Design review of the part built by this model. Coordinates are the model's own, in mm. A direction names the side the tool comes from. Round coordinates to 2 decimals unless told otherwise and drop trailing zeros. Loops run counter-clockwise (first coordinate to the right, second up) from the corner with the lowest first, then second, coordinate; pieces in that order, holes last. Notation, with made-up numbers: (-33.75, -33.5) - (25.25, -33.5) arc R13 cw to (25.25, -13.5) - close; hole circle Ø5 at (-2, 28). An arc over 180 degrees is marked (long way). Answer as CSV lines item,"result". Start each with the question number.
(1) Mouldability with a two-part tool opening along X and no side actions: class faces 1 (the cylindrical face through (-0.46, 57.47, 0.74)), 2 (the cylindrical face through (17.14, 55.1, 0.74)), 3 (the cylindrical face through (0.1, 61.5, 0.7)) as released by +X, released by -X, zero draft, split by the parting line, or undercut.
(2) Consider section C-C (x = -2). Give the boundary of the cut face in (y, z), and give its area (3 significant figures).
(3) Wall thickness on L1, parallel to X at y = 47, z = 0.65; L2, parallel to X at y = -15, z = 1.2; L3, parallel to X at y = 40.5, z = 0.5: over which ranges is each line inside the solid? List them lowest first.
(4) Consider section B-B (y = -15.25). Give the boundary of the cut face in (x, z), and give its area (3 significant figures).
(5) Consider section A-A (y = -52). Give the boundary of the cut face in (x, z).
(6) Consider section D-D (z = 0.55). Count the separate pieces of the cut face and the enclosed holes in it, and give its area (3 significant figures).
(7) For P1, Ø0.8, axis at y = -44, z = 0.5, coming from the +X side, flat-tipped, find the tip position at first contact; note if it passes through.
(8) For faces 4 (the cylindrical face through (14.175, 50.536, 0.74)), 5 (the cylindrical face through (9.86, -55.1, 0.74)), list the 3-axis set-ups (+Z, -Z, +X, -X, +Y, -Y) from which the entire face can be reached by the end or side of a thin tool; tool diameter is ignored.
from build123d import *

# Parameters (mm, degrees)
F0_R     = 1.5
F0_R_2   = 3.5
F1_DEPTH = 1.5
F3_DEPTH = 1.501
F5_DEPTH = 1.501
F6_R     = 5


with BuildPart() as f1:
    # F0 (on Top) → F1 (new body)
    with BuildSketch(Plane.XY):
        with BuildLine():
            Line((-9.233093, 56), (-15, 56))
            ThreePointArc((-15, 56), (-17.12132, 55.12132), (-18, 53))
            Line((-18, 53), (-18, 38.214102))
            Line((-18, 38.214102), (-20, 34.75))
            Line((-20, 34.75), (-20, -34.75))
            Line((-20, -34.75), (-18, -38.214102))
            Line((-18, -38.214102), (-18, -53))
            ThreePointArc((-18, -53), (-17.12132, -55.12132), (-15, -56))
            Line((-15, -56), (-12, -56))
            ThreePointArc((-12, -56), (-9.87868, -55.12132), (-9, -53))
            Line((-9, -53), (-9, -48))
            ThreePointArc((-9, -48), (-6.363961, -41.636039), (0, -39))
            ThreePointArc((0, -39), (6.363961, -41.636039), (9, -48))
            Line((9, -48), (9, -53))
            ThreePointArc((9, -53), (9.87868, -55.12132), (12, -56))
            Line((12, -56), (15, -56))
            ThreePointArc((15, -56), (17.12132, -55.12132), (18, -53))
            Line((18, -53), (18, -38.214102))
            Line((18, -38.214102), (20, -34.75))
            Line((20, -34.75), (20, 34.75))
            Line((20, 34.75), (18, 38.214102))
            Line((18, 38.214102), (18, 53))
            ThreePointArc((18, 53), (17.12132, 55.12132), (15, 56))
            Line((15, 56), (9.233093, 56))
            ThreePointArc((9.233093, 56), (7.697794, 56.422626), (6.595066, 57.571429))
            ThreePointArc((6.595066, 57.571429), (0, 61.5), (-6.595066, 57.571429))
            ThreePointArc((-6.595066, 57.571429), (-7.697794, 56.422626), (-9.233093, 56))
        make_face()
        with Locations((-13.5, -52)):
            Circle(F0_R, mode=Mode.SUBTRACT)
        with Locations((-15.25, -15.25)):
            Circle(F0_R, mode=Mode.SUBTRACT)
        with Locations((13.5, -52)):
            Circle(F0_R, mode=Mode.SUBTRACT)
        with Locations((15.25, -15.25)):
            Circle(F0_R, mode=Mode.SUBTRACT)
        with Locations((-15.25, 15.25)):
            Circle(F0_R, mode=Mode.SUBTRACT)
        with BuildLine():
            Line((-15, 27), (-15, 30))
            ThreePointArc((-15, 30), (-14, 31), (-13, 30))
            Line((-13, 30), (-13, 27))
            ThreePointArc((-13, 27), (-14, 26), (-15, 27))
        make_face(mode=Mode.SUBTRACT)
        with Locations((-14.5, 52)):
            Circle(F0_R, mode=Mode.SUBTRACT)
        with Locations((15.25, 15.25)):
            Circle(F0_R, mode=Mode.SUBTRACT)
        with BuildLine():
            Line((13, 27), (13, 30))
            ThreePointArc((13, 30), (14, 31), (15, 30))
            Line((15, 30), (15, 27))
            ThreePointArc((15, 27), (14, 26), (13, 27))
        make_face(mode=Mode.SUBTRACT)
        with Locations((0, 54)):
            Circle(F0_R_2, mode=Mode.SUBTRACT)
        with Locations((14.5, 52)):
            Circle(F0_R, mode=Mode.SUBTRACT)
    extrude(amount=F1_DEPTH)

    # F2 (on face) → F3 (cut, through all)
    with BuildSketch(Plane.XY.offset(1.5)):
        with BuildLine():
            Line((-14, -41), (-15, -41))
            ThreePointArc((-15, -41), (-15.5, -41.5), (-15, -42))
            Line((-15, -42), (-15, -45))
            ThreePointArc((-15, -45), (-15.5, -45.5), (-15, -46))
            Line((-15, -46), (-14, -46))
            ThreePointArc((-14, -46), (-13.5, -45.5), (-14, -45))
            Line((-14, -45), (-14, -42))
            ThreePointArc((-14, -42), (-13.5, -41.5), (-14, -41))
        make_face()
        with BuildLine():
            Line((-14, -24), (-15, -24))
            ThreePointArc((-15, -24), (-15.5, -24.5), (-15, -25))
            Line((-15, -25), (-15, -28))
            ThreePointArc((-15, -28), (-15.5, -28.5), (-15, -29))
            Line((-15, -29), (-14, -29))
            ThreePointArc((-14, -29), (-13.5, -28.5), (-14, -28))
            Line((-14, -28), (-14, -25))
            ThreePointArc((-14, -25), (-13.5, -24.5), (-14, -24))
        make_face()
        with BuildLine():
            ThreePointArc((15, -29), (15.5, -28.5), (15, -28))
            Line((15, -28), (15, -25))
            ThreePointArc((15, -25), (15.5, -24.5), (15, -24))
            Line((15, -24), (14, -24))
            ThreePointArc((14, -24), (13.5, -24.5), (14, -25))
            Line((14, -25), (14, -28))
            ThreePointArc((14, -28), (13.5, -28.5), (14, -29))
            Line((14, -29), (15, -29))
        make_face()
        with BuildLine():
            Line((14, -46), (15, -46))
            ThreePointArc((15, -46), (15.5, -45.5), (15, -45))
            Line((15, -45), (15, -42))
            ThreePointArc((15, -42), (15.5, -41.5), (15, -41))
            Line((15, -41), (14, -41))
            ThreePointArc((14, -41), (13.5, -41.5), (14, -42))
            Line((14, -42), (14, -45))
            ThreePointArc((14, -45), (13.5, -45.5), (14, -46))
        make_face()
    extrude(amount=-F3_DEPTH, mode=Mode.SUBTRACT)

    # F4 (on face) → F5 (cut, through all)
    with BuildSketch(Plane.XY.offset(1.5)):
        with BuildLine():
            Line((-13.5, 44.5), (-13.5, 47))
            ThreePointArc((-13.5, 47), (-14.5, 48), (-15.5, 47))
            Line((-15.5, 47), (-15.5, 44.5))
            ThreePointArc((-15.5, 44.5), (-14.5, 43.5), (-13.5, 44.5))
        make_face()
        with BuildLine():
            ThreePointArc((15.5, 47), (14.5, 48), (13.5, 47))
            Line((13.5, 47), (13.5, 44.5))
            ThreePointArc((13.5, 44.5), (14.5, 43.5), (15.5, 44.5))
            Line((15.5, 44.5), (15.5, 47))
        make_face()
    extrude(amount=-F5_DEPTH, mode=Mode.SUBTRACT)

    # F6
    f6_edges = [f1.edges().sort_by_distance(p)[0] for p in [
        (-20, 34.75, 0.75),
        (20, 34.75, 0.75),
        (20, -34.75, 0.75),
        (-20, -34.75, 0.75),
        (-18, -38.214102, 0.75),
        (18, -38.214102, 0.75),
        (18, 38.214102, 0.75),
        (-18, 38.214102, 0.75),
    ]]
    fillet(f6_edges, radius=F6_R)


solid = f1.part
Determined:
1,face 1,"undercut"
1,face 2,"released by +X"
1,face 3,"split by the parting line"
2,outline,"(-39.23, 0) - (51.13, 0) - (51.13, 1.5) - (-39.23, 1.5) - close; (56.87, 0) - (61.23, 0) - (61.23, 1.5) - (56.87, 1.5) - close"
2,area,"142 mm^2"
3,L1,"x = -18 to -15.5, -13.5 to 13.5, 15.5 to 18"
3,L2,"x = -20 to -16.73, -13.77 to 13.77, 16.73 to 20"
3,L3,"x = -18 to 18"
4,outline,"(-20, 0) - (-16.75, 0) - (-16.75, 1.5) - (-20, 1.5) - close; (-13.75, 0) - (13.75, 0) - (13.75, 1.5) - (-13.75, 1.5) - close; (16.75, 0) - (20, 0) - (20, 1.5) - (16.75, 1.5) - close"
4,area,"51.0 mm^2"
5,outline,"(-18, 0) - (-15, 0) - (-15, 1.5) - (-18, 1.5) - close; (-12, 0) - (-9, 0) - (-9, 1.5) - (-12, 1.5) - close; (9, 0) - (12, 0) - (12, 1.5) - (9, 1.5) - close; (15, 0) - (18, 0) - (18, 1.5) - (15, 1.5) - close"
6,separate pieces,"1"
6,enclosed holes,"17"
6,area,"3,950 mm^2"
7,P1,"stops at x = 18"
8,face 4,"+Z, -Z"
8,face 5,"+Z, -Z, -Y"
